Can you work these out from the model? Positions are in its coordinate system, mm. A direction names the side the tool comes from. Give positions to 0.01 mm unless a question says otherwise; leave off trailing zeros. Write each loop counter-clockwise with the first axis right and the second up, starting at its lowest first coordinate (ties: lowest second). Pieces come first, ordered by that corner, then holes. Notation, with made-up numbers: (70.5, 17) -> (103.5, 17) arc R8 ccw to (103.5, 28) -> close; hole circle Ø9 at (-15, 50). An arc over 180 degrees is marked (long way). One line per item, written item: value.
from build123d import *

# Parameters (mm, degrees)
SKETCH3_R             = 18.7
BOSS_EXTRUDE1_DEPTH   = 1.2
BOSS_EXTRUDE1_2_DEPTH = 1.2
SKETCH4_R             = 17.5
BOSS_EXTRUDE2_DEPTH   = 4.6
SKETCH5_R             = 18.7
BOSS_EXTRUDE3_DEPTH   = 1.2
SKETCH6_R             = 2
CUT_EXTRUDE1_DEPTH    = 82.193472644
SKETCH7_R             = 6
CUT_EXTRUDE2_DEPTH    = 82.193472644
SWEEP4_START          = 7
SWEEP4_OUTLINE_R      = 10
SWEEP4_DEPTH          = 32
SWEEP4_2_OUTLINE_R    = 6
SWEEP4_2_DEPTH        = 7
SWEEP4_3_OUTLINE_R    = 10
SWEEP4_3_ANGLE        = 180
SKETCH10_R            = 6
CUT_EXTRUDE3_DEPTH    = 7
SKETCH11_R            = 6


with BuildPart() as part:
    # Sketch3 → Boss-Extrude1 (new body)
    with BuildSketch(Plane(origin=(0, 0, 0), x_dir=(1, 0, 0), z_dir=(0, 1, 0))):
        with Locations(Location((0, 0, 0), (0, 0, 270))):
            Circle(SKETCH3_R)
    extrude(amount=BOSS_EXTRUDE1_DEPTH)



with BuildPart() as body_2:
    # Sketch3 → Boss-Extrude1 2 (new body)
    with BuildSketch(Plane(origin=(0, 0, 0), x_dir=(1, 0, 0), z_dir=(0, 1, 0))):
        with Locations(Location((60, 0, 0), (0, 0, 270))):
            Circle(SKETCH3_R)
    extrude(amount=BOSS_EXTRUDE1_2_DEPTH)


with BuildPart() as part_1:
    add(part.part)

    add(body_2.part)  # Boss-Extrude2 merges body 2
    # Sketch4 → Boss-Extrude2 (add)
    with BuildSketch(Plane(origin=(0, 1.2, 0), x_dir=(1, 0, 0), z_dir=(0, 1, 0))):
        with Locations(Location((0, 0, 0), (0, 0, 270))):
            Circle(SKETCH4_R)
        with Locations(Location((60, 0, 0), (0, 0, 270))):
            Circle(SKETCH4_R)
    extrude(amount=BOSS_EXTRUDE2_DEPTH)

    # Sketch5 → Boss-Extrude3 (add)
    with BuildSketch(Plane(origin=(0, 5.8, 0), x_dir=(1, 0, 0), z_dir=(0, 1, 0))):
        with Locations(Location((0, 0, 0), (0, 0, 270))):
            Circle(SKETCH5_R)
        with Locations(Location((60, 0, 0), (0, 0, 270))):
            Circle(SKETCH5_R)
    extrude(amount=BOSS_EXTRUDE3_DEPTH)

    # Sketch6 → Cut-Extrude1 (cut, through all)
    with BuildSketch(Plane(origin=(0, 7, 0), x_dir=(1, 0, 0), z_dir=(0, 1, 0))):
        with Locations(Location((0, 12.441407295, 0), (0, 0, 270))):
            Circle(SKETCH6_R)
        with Locations(Location((12.441407295, 0, 0), (0, 0, 270))):
            Circle(SKETCH6_R)
        with Locations(Location((0, -12.441407295, 0), (0, 0, 270))):
            Circle(SKETCH6_R)
        with Locations(Location((-12.441407295, 0, 0), (0, 0, 270))):
            Circle(SKETCH6_R)
        with Locations(Location((45.570995446, 0, 0), (0, 0, 270))):
            Circle(SKETCH6_R)
        with Locations(Location((60, 14.429004554, 0), (0, 0, 270))):
            Circle(SKETCH6_R)
        with Locations(Location((74.429004554, 0, 0), (0, 0, 270))):
            Circle(SKETCH6_R)
        with Locations(Location((60, -14.429004554, 0), (0, 0, 270))):
            Circle(SKETCH6_R)
    extrude(amount=-CUT_EXTRUDE1_DEPTH, mode=Mode.SUBTRACT)

    # Sketch7 → Cut-Extrude2 (cut, through all)
    with BuildSketch(Plane(origin=(0, 7, 0), x_dir=(1, 0, 0), z_dir=(0, 1, 0))):
        with Locations(Location((0, 0, 0), (0, 0, 270))):
            Circle(SKETCH7_R)
        with Locations(Location((60, 0, 0), (0, 0, 270))):
            Circle(SKETCH7_R)
    extrude(amount=-CUT_EXTRUDE2_DEPTH, mode=Mode.SUBTRACT)

    # Sweep4: read off the stored shape, not the designer's step
    # Sweep4 outline → Sweep4 (add)
    with BuildSketch(Plane(origin=(0, 0, 0), x_dir=(1, 0, 0), z_dir=(0, 1, 0)).offset(SWEEP4_START)):
        with Locations((60, 0)):
            Circle(SWEEP4_OUTLINE_R)
        Circle(SWEEP4_OUTLINE_R)
    extrude(amount=SWEEP4_DEPTH)

    # Sweep4 2 outline → Sweep4 2 (add)
    with BuildSketch(Plane(origin=(0, 0, 0), x_dir=(1, 0, 0), z_dir=(0, 1, 0))):
        with Locations((60, 0)):
            Circle(SWEEP4_2_OUTLINE_R)
    extrude(amount=SWEEP4_2_DEPTH)

    # Sweep4 3 outline → Sweep4 3 (revolve)
    with BuildSketch(Plane(origin=(30, 39, 0), x_dir=(1, 0, 0), z_dir=(0, -1, 0))):
        with Locations((30, 0)):
            Circle(SWEEP4_3_OUTLINE_R)
    revolve(axis=Axis((30, 39, 0), (0, 0, 1)), revolution_arc=SWEEP4_3_ANGLE)

    # Sketch10 → Cut-Extrude3 (cut)
    with BuildSketch(Plane(origin=(0, 0, 0), x_dir=(-1, 0, 0), z_dir=(0, -1, 0))):
        with Locations(Location((-60, 0, 0), (0, 0, 90))):
            Circle(SKETCH10_R)
    extrude(amount=-CUT_EXTRUDE3_DEPTH, mode=Mode.SUBTRACT)

    # Cut-Sweep3: sweep along a path in Sketch12
    with BuildLine(Plane.XY) as cut_sweep3_path:
        Line((0, 7), (0, 40))
        ThreePointArc((0, 40), (30, 70), (60, 40))
        Line((60, 40), (60, 7))
    # Sketch11 → Cut-Sweep3 (sweep, cut)
    with BuildSketch(Plane.XZ.offset(-7)):
        Circle(SKETCH11_R)
    sweep(path=cut_sweep3_path.line, mode=Mode.SUBTRACT)


solid = part_1.part
1) For faces 3 (the face through (78.54, 6.39, -2.43)), 4 (the face through (46, 1.2, 11)), 5 (the face through (76.1, 3.5, 1.1)), which set-ups out of +Z, -Z, +X, -X, +Y, -Y let a thin tool reach every point of the face, with its end or its side?
Answer list:
face 3: -Y
face 4: none
face 5: +Y, -Y
2) If we section it at A-A (y = 26.5): Write out the boundary of the cut face in (x, z), and give its area (3 significant figures).
Answer list:
outline: circle Ø20 at (0, 0); circle Ø20 at (60, 0); hole circle Ø12 at (0, 0); hole circle Ø12 at (60, 0)
area: 402 mm^2
3) I need wall thicknesses on L1, parallel to X at y = 12, z = 0; L2, parallel to Z at x = 0, y = 24; L3, parallel to X at y = 12, z = 1. Which ranges of each line are inside material? Lowest first, please.
Answer list:
L1: x = -10 to -6, 6 to 10, 50 to 54, 66 to 70
L2: z = -10 to -6, 6 to 10
L3: x = -9.95 to -5.92, 5.92 to 9.95, 50.05 to 54.08, 65.92 to 69.95
4) If we section it at B-B (x = 0): State how many separate pieces and enclosed holes the cut face has, and give its area (3 significant figures).
Answer list:
separate pieces: 3
enclosed holes: 0
area: 604 mm^2
5) Will these pins go through, and if not, where does the flat tip stop? pin 1 (1.5 mm diameter, centred on y = 19.5, z = 12.5, fed in from -X); pin 2 (4.5 mm diameter, centred on x = -12.44, z = 0, fed in from +Y); pin 3 (8 mm diameter, centred on y = 52, z = 1, fed in from +X); pin 4 (15.5 mm diameter, centred on x = 60, z = 0, fed in from +Y).
Answer list:
pin 1: passes through
pin 2: stops at y = 7
pin 3: stops at x = 68.96
pin 4: stops at y = 72.24
6) We'd pull the mould along X, two halves only. Please class faces 1 (the face through (52, 7, 8)), 2 (the face through (4.4, 0, -4.4)): released by +X, released by -X, zero draft, split by the parting line, or undercut.
Answer list:
face 1: undercut
face 2: zero draft
